```python
from build123d import *

# Parameters (mm, degrees)
SKETCH1_R           = 100
SKETCH1_R_2         = 1.65
BOSS_EXTRUDE1_DEPTH = 3
SKETCH2_R           = 12.5
CUT_EXTRUDE1_DEPTH  = 4


with BuildPart() as part:
    # Sketch1 → Boss-Extrude1 (new body)
    with BuildSketch(Plane(origin=(0, 0, 0), x_dir=(1, 0, 0), z_dir=(0, 1, 0))):
        Circle(SKETCH1_R)
        with Locations((-87, 0)):
            Circle(SKETCH1_R_2, mode=Mode.SUBTRACT)
        with Locations((-43.5, 75.344210129)):
            Circle(SKETCH1_R_2, mode=Mode.SUBTRACT)
        with Locations((43.5, 75.344210129)):
            Circle(SKETCH1_R_2, mode=Mode.SUBTRACT)
        with Locations((87, 0)):
            Circle(SKETCH1_R_2, mode=Mode.SUBTRACT)
        with Locations((43.5, -75.344210129)):
            Circle(SKETCH1_R_2, mode=Mode.SUBTRACT)
        with Locations((-43.5, -75.344210129)):
            Circle(SKETCH1_R_2, mode=Mode.SUBTRACT)
    extrude(amount=BOSS_EXTRUDE1_DEPTH)

    # Sketch2 → Cut-Extrude1 (cut, through all)
    with BuildSketch(Plane(origin=(0, 3, 0), x_dir=(1, 0, 0), z_dir=(0, 1, 0))):
        Circle(SKETCH2_R)
    extrude(amount=-CUT_EXTRUDE1_DEPTH, mode=Mode.SUBTRACT)


solid = part.part
```
Here's how the part is built. I have some questions about the finished solid (model axes, mm). Round coordinates to 2 decimals unless told otherwise and drop trailing zeros. Write each loop counter-clockwise with the first axis right and the second up, starting at its lowest first coordinate (ties: lowest second). Pieces come first, ordered by that corner, then holes.
Q1. If we section it at D-D on x = -66: Write out the boundary of the cut face in (y, z), plus the area to 3 significant figures.
Q2. If we section it at A-A on x = 0: Write out the boundary of the cut face in (y, z), plus the area to 3 significant figures.
Q3. If we section it at B-B on y = 1.85: Write out the boundary of the cut face in (x, z).
Q4. Will these pins go through, and if not, where does the flat tip stop? P1, Ø5.5, axis at x = 87, z = 0, coming from the -Y side; P2, Ø1, axis at y = 1, z = -24.5, coming from the +X side; P3, Ø1, axis at y = 2.5, z = 26, coming from the +X side.
Q5. Please list where these lines run through material, in increasing order: probe 1 along X at (y, z) = (0.85, 0); probe 2 along Z at (x, y) = (0, 2.8); probe 3 along Z at (x, y) = (-43.5, 2.45).
Q6. If we section it at C-C on z = 28: Write out the boundary of the cut face in (x, y).
Q7. If we mould it in two halves opening along X, with no side actions, what happens to faces 1 (the cylindrical face through (11.923, 1.521, -3.755)), 2 (the flat face through (-1, 0, 21)), 3 (the cylindrical face through (95.38, 1.48, -30.04))? For each: +X half, -X half, draft (parallel to the pull), parting line (faces both ways), or undercut.
Answer below:
1. outline: (0, -75.13) - (3, -75.13) - (3, 75.13) - (0, 75.13) - close
1. area: 451 mm2
2. outline: (0, -100) - (3, -100) - (3, -12.5) - (0, -12.5) - close; (0, 12.5) - (3, 12.5) - (3, 100) - (0, 100) - close
2. area: 525 mm2
3. outline: circle Ø200 at (0, 0); hole circle Ø3.3 at (-87, 0); hole circle Ø3.3 at (-43.5, -75.34); hole circle Ø3.3 at (-43.5, 75.34); hole circle Ø25 at (0, 0); hole circle Ø3.3 at (43.5, -75.34); hole circle Ø3.3 at (43.5, 75.34); hole circle Ø3.3 at (87, 0)
4. P1: stops at y = 0
4. P2: stops at x = 97.08
4. P3: stops at x = 96.69
5. probe 1: x = -100 to -88.65, -85.35 to -12.5, 12.5 to 85.35, 88.65 to 100
5. probe 2: z = -100 to -12.5, 12.5 to 100
5. probe 3: z = -90.04 to -76.99, -73.69 to 73.69, 76.99 to 90.04
6. outline: (-96, 0) - (96, 0) - (96, 3) - (-96, 3) - close
7. face 1: undercut
7. face 2: draft
7. face 3: parting line
